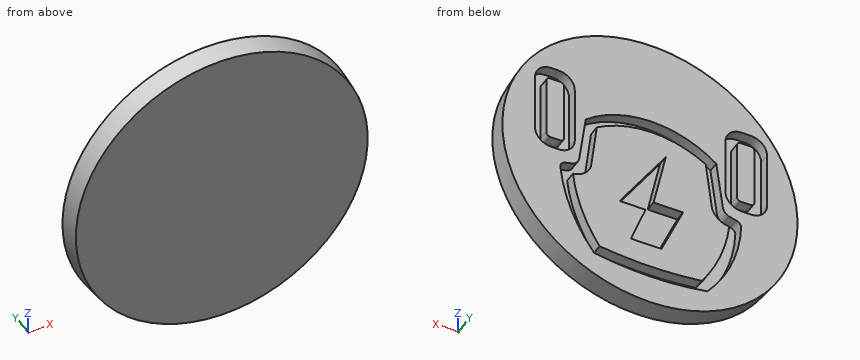
```python
from build123d import *

# Parameters (mm, degrees)
CROQUIS1_R              = 26.25
SALIENTE_EXTRUIR1_DEPTH = 4
CORTAR_EXTRUIR2_DEPTH   = 2
CROQUIS3_R              = 26.75
CROQUIS3_R_2            = 26.25
SALIENTE_EXTRUIR2_DEPTH = 4
CHAFL_N2_SIZE           = 0.3
CHAFL_N2_SIZE_2         = 4


with BuildPart() as part:
    # Croquis1 → Saliente-Extruir1 (new body)
    with BuildSketch(Plane(origin=(0, 0, 0), x_dir=(1, 0, 0), z_dir=(0, 1, 0))):
        with Locations(Location((0, 0, 0), (0, 0, 270))):
            Circle(CROQUIS1_R)
    extrude(amount=SALIENTE_EXTRUIR1_DEPTH)

    # Croquis2 → Cortar-Extruir2 (cut)
    # profile 1 of 4: a face of its own
    with BuildSketch(Plane(origin=(0, 4, 0), x_dir=(1, 0, 0), z_dir=(0, 1, 0))):
        with BuildLine():
            Line((16.577628019, 1.378684251), (17.872942997, 1.378684251))
            ThreePointArc((17.872942997, 1.378684251), (19.958908001, 0.514649256), (20.822942997, -1.571315749))
            Line((20.822942997, -1.571315749), (20.822942997, -12.099082076))
            ThreePointArc((20.822942997, -12.099082076), (19.958908001, -14.18504708), (17.872942997, -15.049082076))
            Line((17.872942997, -15.049082076), (16.577628019, -15.049082076))
            ThreePointArc((16.577628019, -15.049082076), (14.491663014, -14.18504708), (13.627628019, -12.099082076))
            Line((13.627628019, -12.099082076), (13.627628019, -1.571315749))
            ThreePointArc((13.627628019, -1.571315749), (14.491663014, 0.514649256), (16.577628019, 1.378684251))
        make_face()
        with BuildLine():
            ThreePointArc((16.26679092, -0.611177343), (15.771816174, -0.816202597), (15.56679092, -1.311177343))
            Line((15.56679092, -1.311177343), (15.56679092, -12.108932122))
            ThreePointArc((15.56679092, -12.108932122), (15.771816174, -12.603906869), (16.26679092, -12.808932122))
            Line((16.26679092, -12.808932122), (18.08171889, -12.808932122))
            ThreePointArc((18.08171889, -12.808932122), (18.576693636, -12.603906869), (18.78171889, -12.108932122))
            Line((18.78171889, -12.108932122), (18.78171889, -1.311177343))
            ThreePointArc((18.78171889, -1.311177343), (18.576693636, -0.816202597), (18.08171889, -0.611177343))
            Line((18.08171889, -0.611177343), (16.26679092, -0.611177343))
        make_face(mode=Mode.SUBTRACT)
    # profile 2 of 4: a face of its own
    with BuildSketch(Plane(origin=(0, 4, 0), x_dir=(1, 0, 0), z_dir=(0, 1, 0))):
        with BuildLine():
            ThreePointArc((-16.541154267, 4.559666994), (-14.820529985, 13.034857679), (-10.397118387, 20.466064507))
            ThreePointArc((-10.397118387, 20.466064507), (-0.144491455, 21.407214974), (10.108135477, 20.466064507))
            ThreePointArc((10.108135477, 20.466064507), (14.207692764, 13.245645686), (16.196417943, 5.184269249))
            ThreePointArc((16.196417943, 5.184269249), (16.132024065, 4.288372794), (15.452996259, 3.700411684))
            Line((15.452996259, 3.700411684), (14.173141036, 3.380229026))
            ThreePointArc((14.173141036, 3.380229026), (13.270359302, 2.836290622), (12.826889255, 1.880143059))
            Line((12.826889255, 1.880143059), (11.63113204, -6.78360674))
            ThreePointArc((11.63113204, -6.78360674), (-0.193198097, -10.969098115), (-12.017528234, -6.78360674))
            Line((-12.017528234, -6.78360674), (-13.210287359, 1.886657738))
            ThreePointArc((-13.210287359, 1.886657738), (-13.568040347, 2.740473566), (-14.30282929, 3.303566701))
            Line((-14.30282929, 3.303566701), (-15.641463565, 3.64729627))
            ThreePointArc((-15.641463565, 3.64729627), (-16.21669402, 3.979839116), (-16.541154267, 4.559666994))
        make_face()
        with BuildLine():
            ThreePointArc((-9.39054296, 18.667613115), (-0.129607572, 19.310065951), (9.131327816, 18.667613115))
            ThreePointArc((9.131327816, 18.667613115), (12.342092273, 12.334309576), (13.946689107, 5.417300749))
            ThreePointArc((13.946689107, 5.417300749), (11.898739751, 4.524535831), (10.6848875, 2.648985651))
            Line((10.6848875, 2.648985651), (9.622585247, -5.908678465))
            ThreePointArc((9.622585247, -5.908678465), (-0.243319564, -8.757565726), (-10.109224375, -5.908678465))
            Line((-10.109224375, -5.908678465), (-11.267843272, 2.930632851))
            ThreePointArc((-11.267843272, 2.930632851), (-12.439150787, 4.651094628), (-14.374319564, 5.417300749))
            ThreePointArc((-14.374319564, 5.417300749), (-12.712019595, 12.354486023), (-9.39054296, 18.667613115))
        make_face(mode=Mode.SUBTRACT)
    # profile 3 of 4: a face of its own
    with BuildSketch(Plane(origin=(0, 4, 0), x_dir=(1, 0, 0), z_dir=(0, 1, 0))):
        with BuildLine():
            Line((-21.221754159, -1.571315749), (-21.221754159, -12.099082076))
            ThreePointArc((-21.221754159, -12.099082076), (-20.357719163, -14.18504708), (-18.271754159, -15.049082076))
            Line((-18.271754159, -15.049082076), (-16.629915981, -15.049082076))
            ThreePointArc((-16.629915981, -15.049082076), (-14.543950977, -14.18504708), (-13.679915981, -12.099082076))
            Line((-13.679915981, -12.099082076), (-13.679915981, -1.571315749))
            ThreePointArc((-13.679915981, -1.571315749), (-14.543950977, 0.514649256), (-16.629915981, 1.378684251))
            Line((-16.629915981, 1.378684251), (-18.271754159, 1.378684251))
            ThreePointArc((-18.271754159, 1.378684251), (-20.357719163, 0.514649256), (-21.221754159, -1.571315749))
        make_face()
        with BuildLine():
            ThreePointArc((-16.470722605, -12.808932122), (-15.975747858, -12.603906869), (-15.770722605, -12.108932122))
            Line((-15.770722605, -12.108932122), (-15.770722605, -1.311177343))
            ThreePointArc((-15.770722605, -1.311177343), (-15.975747858, -0.816202597), (-16.470722605, -0.611177343))
            Line((-16.470722605, -0.611177343), (-18.213155179, -0.611177343))
            ThreePointArc((-18.213155179, -0.611177343), (-18.708129925, -0.816202597), (-18.913155179, -1.311177343))
            Line((-18.913155179, -1.311177343), (-18.913155179, -12.108932122))
            ThreePointArc((-18.913155179, -12.108932122), (-18.708129925, -12.603906869), (-18.213155179, -12.808932122))
            Line((-18.213155179, -12.808932122), (-16.470722605, -12.808932122))
        make_face(mode=Mode.SUBTRACT)
    # profile 4 of 4: a face of its own
    with BuildSketch(Plane(origin=(0, 4, 0), x_dir=(1, 0, 0), z_dir=(0, 1, 0))):
        Polygon((5.502535459, 7.821900935), (0.799555116, 7.821900935), (3.451735919, 14.875951975), (-2.071830813, 14.875951975), (-6.012416606, 5.739731652), (-0.66220899, 5.739731652), (-2.874648277, -4.596906534), align=None)
    extrude(amount=-CORTAR_EXTRUIR2_DEPTH, mode=Mode.SUBTRACT)

    # Croquis3 → Saliente-Extruir2 (add)
    with BuildSketch(Plane.XZ):
        with Locations(Location((0, 0, 0), (0, 0, 270))):
            Circle(CROQUIS3_R)
        Circle(CROQUIS3_R_2, mode=Mode.SUBTRACT)
    extrude(amount=-SALIENTE_EXTRUIR2_DEPTH)

    # Chaflán2
    # the kernel refuses this chamfer: 4, 0.3 mm, written as the material it takes off along each edge
    with BuildSketch(Plane(origin=(0, 0, 0), x_dir=(0, 0, -1), z_dir=(-1, 0, 0))) as chafl_n2_piece_1:
        Polygon((26.75 - CHAFL_N2_SIZE, 0), (26.75, -CHAFL_N2_SIZE_2), (26.75, 0), align=None)
    revolve(axis=Axis((0, 0, 0), (0, -1, 0)), mode=Mode.SUBTRACT)


solid = part.part
```
Geometry check sheet. Reference: the model listing, model coordinates, mm. Coordinates: 2 decimals unless noted, no trailing zeros. Order: outer loops, then holes, each group sorted by start corner. A loop starts at its lowest first (then second) coordinate and runs counter-clockwise, first axis right, second up.
Item 1: Section check B-B (z = 0). Enter the section's corners in (x, y).
Item 2: Scan lines: line 1 along X through (y, z) = (3.35, -7.5); line 2 along X through (y, z) = (2.05, -10.5); line 3 along Z through (x, y) = (8.5, 3). Record each from-to range of solid material in increasing order.
Item 3: Depth check by flat-ended pin: pin 1 (1.5 mm diameter, centred on x = -2.5, y = 3.5, fed in from -Z); pin 2 (2 mm diameter, centred on y = 3, z = 5, fed in from -X); pin 3 (0.6 mm diameter, centred on x = 17.5, y = 3.5, fed in from +Z). Enter the tip coordinate at first touch or a pass-through.
Item 4: Section check A-A (y = 2.7). Count the separate pieces of the cut face and the enclosed holes in it, plus the area to 3 significant figures.
Item 5: Section check C-C (x = 0). Enter the section's corners in (y, z), plus the area to 3 significant figures.
Check sheet entries:
1. outline: (-26.75, 4) - (-26.45, 0) - (26.45, 0) - (26.75, 4) - (20.37, 4) - (20.37, 2) - (14.08, 2) - (14.08, 4) - (12.57, 4) - (12.57, 2) - (10.36, 2) - (10.36, 4) - (0.23, 4) - (0.23, 2) - (-1.89, 2) - (-1.89, 4) - (-10.88, 4) - (-10.88, 2) - (-12.95, 2) - (-12.95, 4) - (-14.13, 4) - (-14.13, 2) - (-20.77, 2) - (-20.77, 4) - close
2. line 1: x = -25.63 to -16.28, -14.07 to -5.25, 5.29 to 13.65, 15.86 to 25.63
2. line 2: x = -24.44 to -15.65, -13.34 to -3.96, 1.81 to 12.94, 15.15 to 24.44
2. line 3: z = -25.28 to -20.74, -18.75 to 6.56, 8.84 to 25.28
3. pin 1: stops at z = -26.68
3. pin 2: stops at x = -26.39
3. pin 3: stops at z = 20.44
4. separate pieces: 4
4. enclosed holes: 4
4. area: 1,780 mm2
5. outline: (0, -26.45) - (4, -26.75) - (4, -21.41) - (2, -21.41) - (2, -19.31) - (4, -19.31) - (4, -14.88) - (2, -14.88) - (2, 0.34) - (4, 0.34) - (4, 8.76) - (2, 8.76) - (2, 10.97) - (4, 10.97) - (4, 26.75) - (0, 26.45) - close
5. area: 174 mm2
